The figure shows three views and two pictorial views of one solid part (mm, origin at its lowest corner). Answer the questions. A direction names the side the tool comes from. Round coordinates to 2 decimals unless told otherwise and drop trailing zeros. Order: outer loops, then holes, each group sorted by start corner. A loop starts at its lowest first (then second) coordinate and runs counter-clockwise, first axis right, second up. Notation, with made-up numbers: (26.25, 23.5) -> (52.25, 23.5) arc R13 ccw to (52.25, 39.5) -> close; hole circle Ø1 at (-38, 6). An arc over 180 degrees is marked (long way). Return JSON: item names as keys, results as strings. Group by question number.
(1) Consider line 1 (Z direction, x = 46, y = 2.7) (1 decimal); line 2 (Z direction, x = 45.5, y = 3) (1 decimal); line 3 (X direction, y = 0.4, z = 44.5) (1 decimal). Determine where each line is inside the solid, lowest interval first. Write a range as [from, to].
(2) This flat-tipped pin is pushed along its axis until it touches: pin 1 (2.5 mm diameter, centred on x = 5.55, z = 45.25, fed in from +Y). Where does it stop, or does it pass through?
(3) The part is cut by section B-B (y = 2.5). Count the separate pieces of the cut face and the enclosed holes in it, plus the area to 3 significant figures.
(4) The part is cut by section D-D (x = 38.5). Determine the outline of the cut face in (y, z) (1 decimal).
(5) Which of the six approach directions +Z, -Z, +X, -X, +Y, -Y give full straight-line access (tool end or side, diameter ignored) to the marked faces 1 and 2?
(6) The part is cut by section A-A (x = 25.4). Determine the outline of the cut face in (y, z) (1 decimal).
(7) The part is cut by section C-C (z = 25.4). Determine the outline of the cut face in (x, y) (1 decimal).
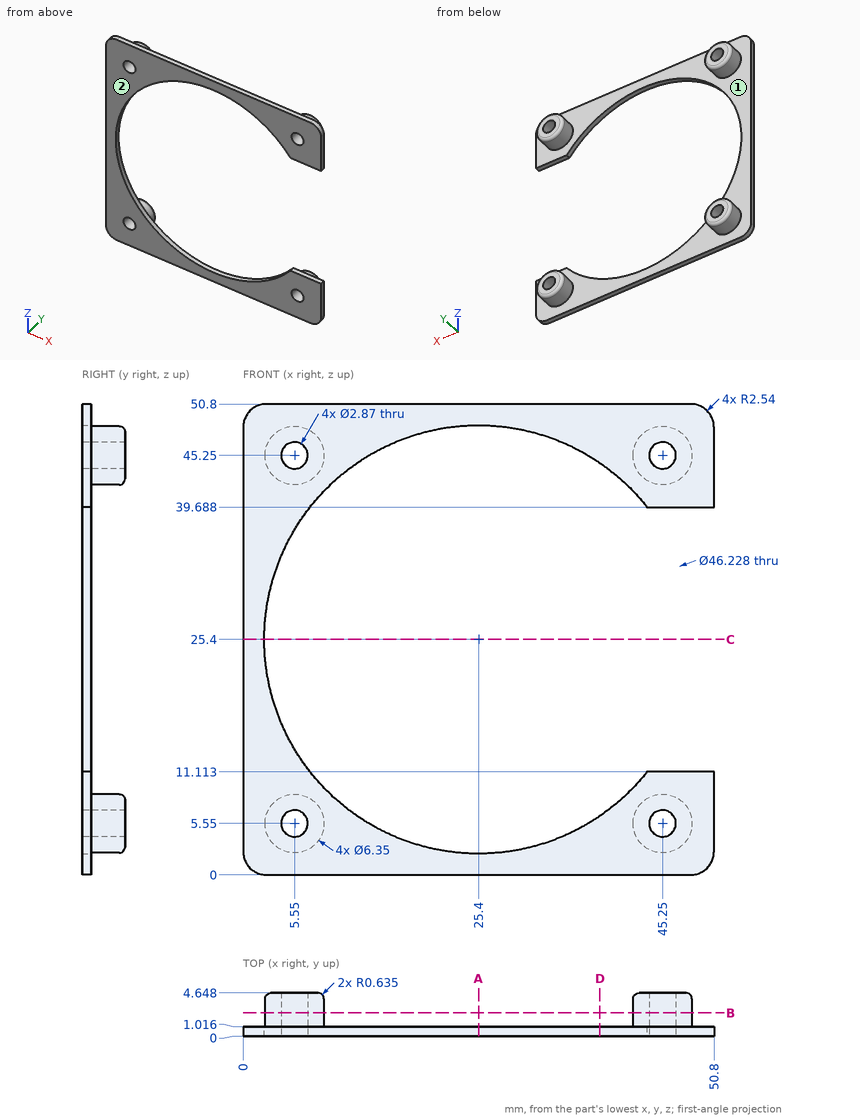
Answer below:
{
 "1": {"line 1": "z = [2.5, 4.3], [6.8, 8.6], [42.2, 44], [46.5, 48.3]", "line 2": "z = [2.4, 4.1], [7, 8.7], [42.1, 43.8], [46.7, 48.4]", "line 3": "x = [0, 4.3], [6.8, 12.4], [38.4, 44], [46.5, 50.8]"},
 "2": {"pin 1": "passes through"},
 "3": {"separate pieces": "4", "enclosed holes": "4", "area": "101 mm²"},
 "4": {"outline": "(0, 0) -> (1, 0) -> (1, 6.4) -> (0, 6.4) -> close; (0, 44.4) -> (1, 44.4) -> (1, 50.8) -> (0, 50.8) -> close"},
 "5": {"face 1": "+Y", "face 2": "+Z, -Z, +X, -X, -Y"},
 "6": {"outline": "(0, 0) -> (1, 0) -> (1, 2.3) -> (0, 2.3) -> close; (0, 48.5) -> (1, 48.5) -> (1, 50.8) -> (0, 50.8) -> close"},
 "7": {"outline": "(0, 0) -> (2.3, 0) -> (2.3, 1) -> (0, 1) -> close"}
}
